Verification items for the finished model (mm, model axes). A direction names the side the tool comes from. Give positions to 0.01 mm unless a question says otherwise; leave off trailing zeros. Loops run counter-clockwise (first coordinate to the right, second up) from the corner with the lowest first, then second, coordinate; pieces in that order, holes last. Notation, with made-up numbers: (5.5, 6.25) - (21.5, 6.25) arc R23 cw to (21.5, 24.25) - close; hole circle Ø3 at (-12.5, 35.5). An arc over 180 degrees is marked (long way). Use one line per item in the form item = value.
Autodesk Fusion 360 part; units mm, degrees
sketch "Sketch1" plane through (0, 0, 0) normal (0, 1, 0) x (1, 0, 0)
  line L0 (-51.7543, 55.7578) -> (88.2457, 55.7578)
  line L1 (88.2457, 55.7578) -> (88.2457, -54.2422)
  line L2 (88.2457, -54.2422) -> (-51.7543, -54.2422)
  line L3 (-51.7543, -54.2422) -> (-51.7543, 55.7578)
  line L4 (-34.6167, 55.7578) -> (-34.6167, 25.7578)
  line L5 (-4.6987, -54.2422) -> (-4.6987, -24.2422)
  line L6 (-51.7543, -24.2422) -> (88.2457, -24.2422)
  line L7 (-51.7543, 25.7578) -> (88.2457, 25.7578)
  line L8 (62.4536, 19.2578) -> (83.4536, 19.2578)
  line L9 (83.4536, 19.2578) -> (83.4536, -17.7422)
  line L10 (83.4536, -17.7422) -> (62.4536, -17.7422)
  line L11 (62.4536, -17.7422) -> (62.4536, 19.2578)
  line L12 (28.1038, -13.9922) -> (12.5038, -13.9922)
  line L13 (12.5038, -13.9922) -> (12.5038, 15.5078)
  circle A0 centre (20.3038, 0.7578) radius 6
  line L14 (12.5038, -13.9922) -> (28.1038, 15.5078)
  line L15 (12.5038, 15.5078) -> (28.1038, -13.9922)
  line L16 (12.5038, 15.5078) -> (28.1038, 15.5078)
  line L17 (28.1038, 15.5078) -> (28.1038, -13.9922)
  line L18 (-7.8, 15.5078) -> (7.8, 15.5078)
  line L19 (-7.8, 15.5078) -> (7.8, -13.9922)
  circle A1 centre (0, 0.7578) radius 6
  line L20 (-7.8, -13.9922) -> (7.8, 15.5078)
  line L21 (-7.8, -13.9922) -> (-7.8, 15.5078)
  line L22 (7.8, 15.5078) -> (7.8, -13.9922)
  line L23 (7.8, -13.9922) -> (-7.8, -13.9922)
  line L24 (-51.7543, 0.7578) -> (88.2457, 0.7578)
  circle A2 centre (36.5574, 13.2578) radius 5
  line L25 (88.2457, 25.7578) -> (88.2457, 0.7578)
  line L26 (88.2457, 0.7578) -> (88.2457, -24.2422)
  line L27 (88.2457, 13.2578) -> (-51.7543, 13.2578)
  circle A3 centre (51.09, 13.2578) radius 5
  circle A4 centre (44.5885, -6.7531) radius 9.5
  circle A5 centre (-29.6042, 0.7578) radius 11.5
  point P0 (20.3038, 0.7578)
  point P1 (35.7195, -1.6286)
  point P2 (0, 0.7578)
  point P3 (-51.7543, 0.7578)
  point P4 (83.4536, 0.7578)
  point P5 (88.2457, 13.2578)
  point P6 (88.2457, -11.7422)
  dimension "d1" = 140
  dimension "d2" = 110
  dimension "d3" = 30
  dimension "d4" = 30
  dimension "d5" = 21
  dimension "d6" = 37
  dimension "d10" = 15.6
  dimension "d11" = 29.5
  dimension "d12" = 12
  dimension "d16" = 15.6
  dimension "d17" = 29.5
  dimension "d18" = 12
  dimension "d19" = 10
  dimension "d20" = 10
  dimension "d21" = 19
  dimension "d22" = 23
extrude "Extrude1" add sketch "Sketch1" along normal blind 3 contours L0 L3 L4 L7 | L0 L1 L4 L7 | L1 L3 L7 L8 L9 L11 L13 L16 L17 L18 L21 L22 A2 L25 L27 A3 | L3 L21 L24 L27 A5 | L1 L3 L6 L9 L10 L11 L12 L13 L17 L21 L22 L23 L24 L26 A4 A5 | L19 A1 L21 L24 L27 | L19 L21 L27 | L1 L9 L24 L25 L27 | L2 L3 L5 L6 | A1 L20 L21 L24 | L18 L19 L20 L27 | L19 A1 L20 L27 | L1 L2 L5 L6 | L19 A1 L20 L23 | L20 L22 L27 | A1 L20 L22 L24 L27 | L11 L17 L24 A2 L27 A3 A4 | L19 A1 L22 L24 | L13 L22 L24 L27 | L13 A0 L15 L24 L27 | L13 L15 L27 | L13 A0 L14 L24 | L14 L15 L16 L27 | A0 L14 L15 L27 | L12 A0 L14 L15 | L14 L17 L27 | A0 L14 L17 L24 L27 | A0 L15 L17 L24
sketch "Sketch2" plane through (0, 3, 0) normal (0, 1, 0) x (-1, 0, 0)
  line L0 (-83.4536, 17.7422) -> (-62.4536, 17.7422)
  line L1 (-62.4536, 17.7422) -> (-62.4536, -19.2578)
  line L2 (-62.4536, -19.2578) -> (-83.4536, -19.2578)
  line L3 (-83.4536, -19.2578) -> (-83.4536, 17.7422)
  circle A0 centre (-36.5574, -13.2578) radius 5
  circle A1 centre (-20.3038, -0.7578) radius 6
  circle A2 centre (-51.09, -13.2578) radius 5
  circle A3 centre (0, -0.7578) radius 6
  circle A4 centre (-44.5885, 6.7531) radius 9.5
  circle A5 centre (29.6042, -0.7578) radius 11.5
  line L4 (-88.2457, 54.2422) -> (-88.2457, -55.7578)
  line L5 (-88.2457, -55.7578) -> (51.7543, -55.7578)
  line L6 (51.7543, -55.7578) -> (51.7543, 54.2422)
  line L7 (51.7543, 54.2422) -> (-88.2457, 54.2422)
  line L8 (-17.1333, -55.7578) -> (-17.1333, -40.7578)
  line L9 (51.7543, -40.7578) -> (-88.2457, -40.7578)
  line L10 (-18.2457, 54.2422) -> (-18.2457, 39.2422)
  line L11 (51.7543, 39.2422) -> (-88.2457, 39.2422)
  line L12 (51.7543, -40.7578) -> (36.7543, -40.7578)
  line L13 (-88.2457, -40.7578) -> (-73.2457, -40.7578)
  line L14 (51.7543, 39.2422) -> (36.7543, 39.2422)
  line L15 (-88.2457, 39.2422) -> (-73.2457, 39.2422)
  point P0 (36.7543, -40.7578)
  point P1 (36.7543, 39.2422)
  point P2 (-73.2457, 39.2422)
  point P3 (-73.2457, -40.7578)
  dimension "d25" = 15
  dimension "d26" = 15
  dimension "d27" = 15
  dimension "d28" = 15
  dimension "d29" = 15
  dimension "d30" = 15
hole "Hole1" at (-36.7543, 3, -40.7578) at (-36.7543, 3, 39.2422) at (73.2457, 3, -40.7578) at (73.2457, 3, 39.2422) direction (0, -1, 0) diameter 4.8 depth 15 tip angle 180
1. Draft check along Z on faces 1 (the cylindrical face through (-18.635, 1.479, 2.696)), 2 (the cylindrical face through (-5.994, 1.479, -0.494)), 3 (the flat face through (88.246, 1, -2)), 4 (the flat face through (17, 1, -55.758)). Enter one of: released by +Z, released by -Z, zero draft, split by the parting line, or undercut.
Result set:
face_1 = undercut
face_2 = undercut
face_3 = zero draft
face_4 = released by -Z
2. Tool access check on faces 5 (the flat face through (62.454, 1, 0)), 6 (the flat face through (17, 3, -14)). Record the directions out of +Z, -Z, +X, -X, +Y, -Y that give a thin tool (end or side, any length) a straight path to the whole face; none if there is none.
Result set:
face_5 = +Y, -Y
face_6 = +Z, -Z, +X, -X, +Y
3. Depth check by flat-ended pin: pin 1 Ø20.5 at (x, z) = (-29.6, -0.76) entering from +Y. Enter the tip coordinate at first touch or a pass-through.
Result set:
pin_1 = through
4. Section check C-C, the plane x = 51.09. Record the cut outline in (y, z), then the cut area to 3 significant figures.
Result set:
outline = (0, -55.76) - (3, -55.76) - (3, -18.26) - (0, -18.26) - close; (0, -8.26) - (3, -8.26) - (3, -0.17) - (0, -0.17) - close; (0, 13.68) - (3, 13.68) - (3, 54.24) - (0, 54.24) - close
area = 258 mm²
5. Scan lines: probe 1 along X at (y, z) = (1.6, 39.5); probe 2 along X at (y, z) = (0.25, 41); probe 3 along Z at (x, y) = (51.09, 1). Record each from-to range of solid material in increasing order.
Result set:
probe_1 = -51.75 to -39.14, -34.37 to 70.86, 75.63 to 88.25
probe_2 = -51.75 to -38.39, -35.12 to 71.61, 74.88 to 88.25
probe_3 = -55.76 to -18.26, -8.26 to -0.17, 13.68 to 54.24
6. Section check D-D, the plane y = 0.45. State how many separate pieces and enclosed holes the cut face has, then the cut area to 3 significant figures.
Result set:
separate_pieces = 1
enclosed_holes = 11
area = 13,500 mm²
7. Section check B-B, the plane z = 3. Record the cut outline in (x, y).
Result set:
outline = (-51.75, 0) - (-40.47, 0) - (-40.47, 3) - (-51.75, 3) - close; (-18.74, 0) - (-4.68, 0) - (-4.68, 3) - (-18.74, 3) - close; (4.68, 0) - (15.63, 0) - (15.63, 3) - (4.68, 3) - close; (24.98, 0) - (35.86, 0) - (35.86, 3) - (24.98, 3) - close; (53.32, 0) - (62.45, 0) - (62.45, 3) - (53.32, 3) - close; (83.45, 0) - (88.25, 0) - (88.25, 3) - (83.45, 3) - close
8. Section check A-A, the plane x = 0. Record the cut outline in (y, z).
Result set:
outline = (0, -55.76) - (3, -55.76) - (3, -6.76) - (0, -6.76) - close; (0, 5.24) - (3, 5.24) - (3, 54.24) - (0, 54.24) - close
